Here's how the part is built. I have some questions about the finished solid (model axes, mm). Coordinates: 2 decimals unless noted, no trailing zeros. Use one line per item in the form item = value. Start each with the question number.
(1) Will these pins go through, and if not, where does the flat tip stop? P1, Ø1.5, axis at x = -18.5, z = 10.5, coming from the -Y side; P2, Ø3, axis at y = -15.5, z = 19, coming from the +X side; P3, Ø1, axis at y = -15, z = 13.5, coming from the -X side.
(2) Please list where these lines run through material, in increasing order: L1, parallel to X at y = -9, z = 12 (3 decimals); L2, parallel to Y at x = -33, z = 14; L3, parallel to Z at x = -6.5, y = -1.5.
(3) Thinking about a two-plate mould opening in Z: for faces 1 (the conical face through (-36.52, -17.86, 23.39)), 2 (the conical face through (-2.544, 0.289, 11.841)), 3 (the conical face through (-9.29, 2.02, 0.22)), which applies, +Z half, -Z half, draft (parallel to the pull), parting line (faces both ways), or undercut?
```python
from build123d import *

# Parameters (mm, degrees)
F2_T = -2.54
F3_R = 5.08
F4_R = 5.08


with BuildPart() as f1:
    # F0 (on Front) → F1 (revolve)
    with BuildSketch(Plane.XZ):
        Polygon((-38.710538, 0), (0, 0), (-34.087466, 34.087466), (-45.367766, 19.108707), align=None)
    revolve(axis=Axis((-17.043733, 0, 17.043733), (0.707107, 0, -0.707107)))

    # F2
    f2_openings = [f1.faces().sort_by_distance(p)[0] for p in [
        (-26.598087, 0, 39.727616),
    ]]
    offset(amount=F2_T, openings=f2_openings)

    # F3
    f3_edges = [f1.edges().sort_by_distance(p)[0] for p in [
        (-19.108707, 0, 45.367766),
    ]]
    fillet(f3_edges, radius=F3_R)

    # F4
    f4_edges = [f1.edges().sort_by_distance(p)[0] for p in [
        (0, 0, 38.710538),
    ]]
    fillet(f4_edges, radius=F4_R)


solid = f1.part
```
Answer:
q1.P1 = -20.52
q1.P2 = -5.09
q1.P3 = -38.48
q2.L1 = -41.096 to -38.229, -6.821 to -3.375
q2.L2 = -20.54 to -17.06, 17.06 to 20.54
q2.L3 = 0.17 to 2.82, 38.24 to 40.93
q3.face_1 = parting line
q3.face_2 = undercut
q3.face_3 = -Z half
